```python
from build123d import *

# Parameters (mm, degrees)
F0_W     = 70
F0_H     = 70
F1_DEPTH = 70
F2_W     = 50
F2_H     = 40
F3_DEPTH = 50
F4_W     = 40
F4_H     = 40
F5_DEPTH = 30.001
F6_R     = 20
F7_W     = 20
F7_H     = 40
F8_DEPTH = 20.001
F9_SIZE  = 10


with BuildPart() as f1:
    # F0 (on Top) → F1 (new body)
    with BuildSketch(Plane.XY):
        with Locations((35, 35)):
            Rectangle(F0_W, F0_H)
    extrude(amount=F1_DEPTH)

    # F2 (on face) → F3 (cut)
    with BuildSketch(Plane.XY.offset(70)):
        with Locations((25, 20)):
            Rectangle(F2_W, F2_H)
    extrude(amount=-F3_DEPTH, mode=Mode.SUBTRACT)

    # F4 (on face) → F5 (cut, through all)
    with BuildSketch(Plane.XZ.offset(-40)):
        with Locations((20, 50)):
            Rectangle(F4_W, F4_H)
    extrude(amount=-F5_DEPTH, mode=Mode.SUBTRACT)

    # F6
    f6_edges = [f1.edges().sort_by_distance(p)[0] for p in [
        (40, 55, 30),
    ]]
    fillet(f6_edges, radius=F6_R)

    # F7 (on face) → F8 (cut, through all)
    with BuildSketch(Plane(origin=(50, 0, 0), x_dir=(0, -1, 0), z_dir=(-1, 0, 0))):
        with Locations((-10, 50)):
            Rectangle(F7_W, F7_H)
    extrude(amount=-F8_DEPTH, mode=Mode.SUBTRACT)

    # F9
    f9_edges = [f1.edges().sort_by_distance(p)[0] for p in [
        (50, 20, 20),
    ]]
    chamfer(f9_edges, length=F9_SIZE)


solid = f1.part
```
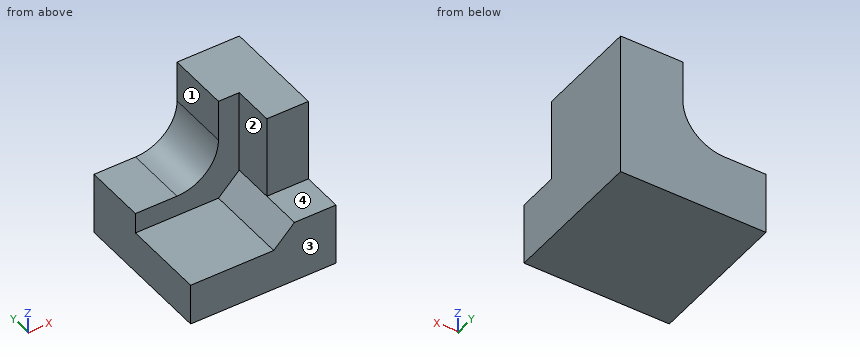
Check sheet for the modelled part. Datum: model origin and axes. Units: mm. Face numbers are marked on the shaded views. A direction names the side the tool comes from. Coordinates: 2 decimals unless noted, no trailing zeros. Loops run counter-clockwise (first coordinate to the right, second up) from the corner with the lowest first, then second, coordinate; pieces in that order, holes last.
1) Access from +Z, -Z, +X, -X, +Y, -Y to the whole of each face (thin tool, end or side, straight path). Record for the marked faces 1, 2, 3 and 4.
2) Material ranges on probe 1 along Y at (x, z) = (9, 28); probe 2 along Z at (x, y) = (23.5, 13); probe 3 along X at (y, z) = (41.5, 36), recorded low to high.
3) Sectioned sample at A-A (y = 36). Record the boundary of the cut face in (x, z), and give its area (3 significant figures).
4) Gauge pin test, flat ends, axial feed: pin 1 (10 mm diameter, centred on y = 50, z = 55, fed in from -X); pin 2 (22 mm diameter, centred on x = 59.5, y = 6, fed in from +Z); pin 3 (5 mm diameter, centred on x = 39.5, z = 45.5, fed in from -Y); pin 4 (12 mm diameter, centred on x = 11, y = 43, fed in from -Z). Record the tip position at first contact, or that the pin passes through.
5) Sectioned sample at B-B (z = 54.5). Record the boundary of the cut face in (x, y).
6) Sectioned sample at C-C (x = 41). Record the boundary of the cut face in (y, z).
Check sheet entries:
1. face 1: +Z, -X, +Y, -Y
1. face 2: +Z, -X, -Y
1. face 3: +Z, -Z, +X, -X, -Y
1. face 4: +Z, +X, -X, -Y
2. probe 1: y = 40 to 70
2. probe 2: z = 0 to 20
2. probe 3: x = 34.28 to 70
3. outline: (0, 0) - (70, 0) - (70, 70) - (50, 70) - (50, 30) - (40, 20) - (0, 20) - close
3. area: 2,450 mm2
4. pin 1: stops at x = 40
4. pin 2: stops at z = 30
4. pin 3: stops at y = 40
4. pin 4: stops at z = 0
5. outline: (40, 40) - (50, 40) - (50, 20) - (70, 20) - (70, 70) - (40, 70) - close
6. outline: (0, 0) - (70, 0) - (70, 70) - (40, 70) - (40, 21) - (0, 21) - close
